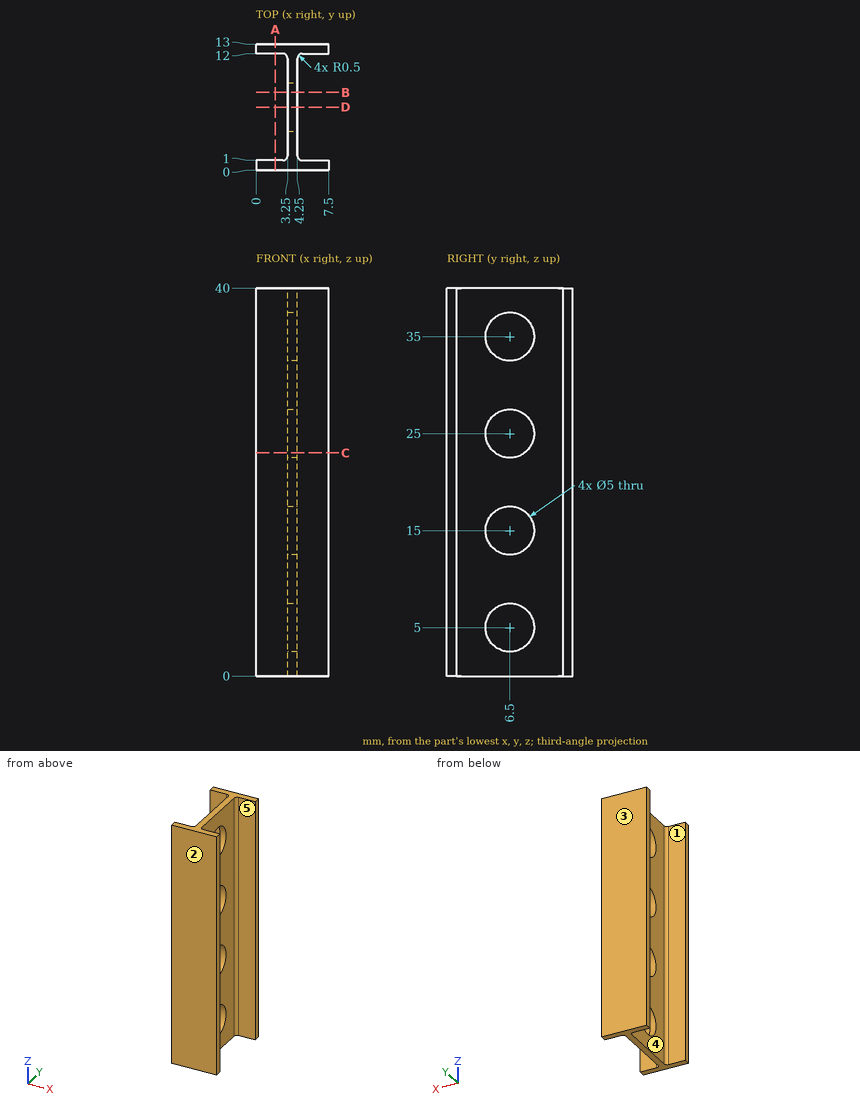
For this review, use the dimensioned drawing (mm, ordinates from the lowest corner) and the shaded views. A direction names the side the tool comes from. Round coordinates to 2 decimals unless told otherwise and drop trailing zeros. Loops run counter-clockwise (first coordinate to the right, second up) from the corner with the lowest first, then second, coordinate; pieces in that order, holes last. Notation, with made-up numbers: M -30.75,-17 L 26.25,-17 A19 ccw 26.25,-13 Z; hole C 12,37.5 d11. An arc over 180 degrees is marked long. Answer as a JSON object with one key per item and string values.
(1) To check wall thickness, follow line 1 along Z through (x, y) = (3.85, 6.5); line 2 along Y through (x, z) = (3.65, 35); line 3 along Y through (x, z) = (6, 29). State the ranges of each line that lie inside material, in increasing order.
Resolved:
{"line 1": "0 to 2.5, 7.5 to 12.5, 17.5 to 22.5, 27.5 to 32.5, 37.5 to 40", "line 2": "0 to 4, 9 to 13", "line 3": "0 to 1, 12 to 13"}
(2) Draft analysis for pull direction Y (two halves, no side actions). For the marked faces 1, 2 and 3, state which applies: released by +Y, released by -Y, zero draft, split by the parting line, or undercut.
Resolved:
{"face 1": "undercut", "face 2": "released by -Y", "face 3": "released by +Y"}
(3) Tool access review of the marked faces 4 and 5: name each direction out of +Z, -Z, +X, -X, +Y, -Y from which nothing blocks a thin tool from reaching the whole face with its end or side.
Resolved:
{"face 4": "+Z, -Z, -X", "face 5": "+Z, -Z, +X"}
(4) Clearance check with flat-ended pins moving along their axes: P1, Ø4, axis at y = 6.5, z = 15, coming from the -X side; P2, Ø1.5, axis at y = 10, z = 10, coming from the +X side; P3, Ø5, axis at y = 5, z = 11.5, coming from the -X side; P4, Ø3, axis at x = 3.5, z = 11.5, coming from the -Y side. State where each tip first meets the part, or that it passes through.
Resolved:
{"P1": "through", "P2": "x = 4.25", "P3": "x = 3.25", "P4": "y = 0"}
(5) Take a section at C-C on z = 23. Give the boundary of the cut face in (x, y), and give its area (3 significant figures).
Resolved:
{"outline": "M 0,0 L 7.5,0 L 7.5,1 L 4.75,1 A0.5 cw 4.25,1.5 L 4.25,5 L 3.25,5 L 3.25,1.5 A0.5 cw 2.75,1 L 0,1 Z; M 0,12 L 2.75,12 A0.5 cw 3.25,11.5 L 3.25,8 L 4.25,8 L 4.25,11.5 A0.5 cw 4.75,12 L 7.5,12 L 7.5,13 L 0,13 Z", "area": "23.2 mm²"}
(6) Take a section at A-A on x = 2. Give the boundary of the cut face in (y, z).
Resolved:
{"outline": "M 0,0 L 1,0 L 1,40 L 0,40 Z; M 12,0 L 13,0 L 13,40 L 12,40 Z"}
(7) Take a section at B-B on y = 8. Give the boundary of the cut face in (x, z).
Resolved:
{"outline": "M 3.25,0 L 4.25,0 L 4.25,3 L 3.25,3 Z; M 3.25,7 L 4.25,7 L 4.25,13 L 3.25,13 Z; M 3.25,17 L 4.25,17 L 4.25,23 L 3.25,23 Z; M 3.25,27 L 4.25,27 L 4.25,33 L 3.25,33 Z; M 3.25,37 L 4.25,37 L 4.25,40 L 3.25,40 Z"}
(8) Take a section at D-D on y = 6.5. Give the boundary of the cut face in (x, z).
Resolved:
{"outline": "M 3.25,0 L 4.25,0 L 4.25,2.5 L 3.25,2.5 Z; M 3.25,7.5 L 4.25,7.5 L 4.25,12.5 L 3.25,12.5 Z; M 3.25,17.5 L 4.25,17.5 L 4.25,22.5 L 3.25,22.5 Z; M 3.25,27.5 L 4.25,27.5 L 4.25,32.5 L 3.25,32.5 Z; M 3.25,37.5 L 4.25,37.5 L 4.25,40 L 3.25,40 Z"}
